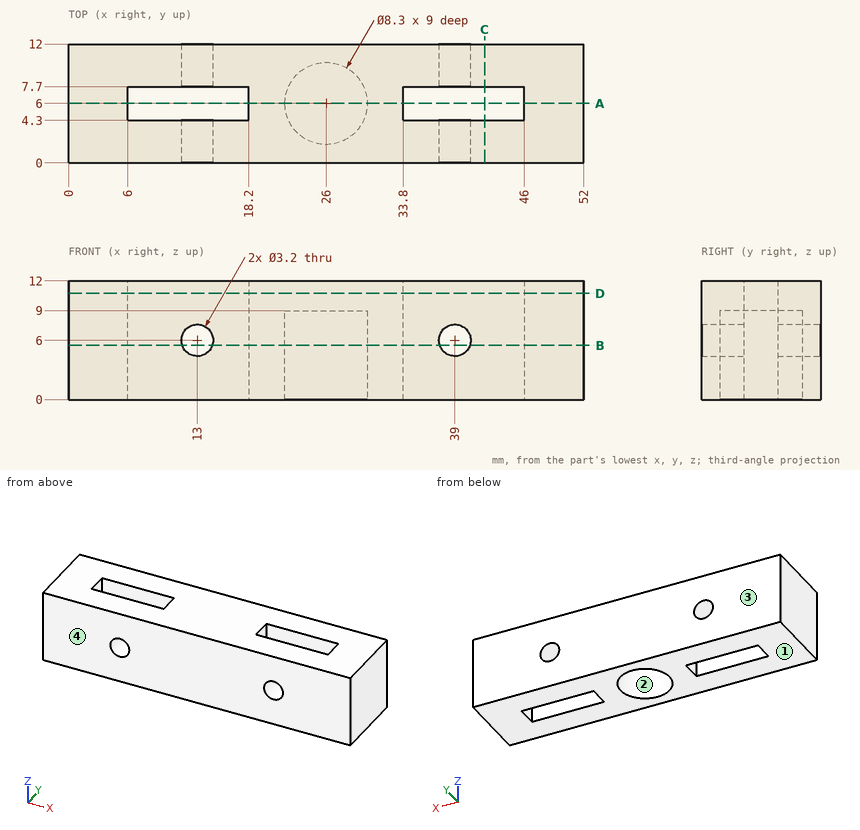
Input: dimensioned drawing with shaded views. Units: mm. Origin: part minimum x, y, z. Round coordinates to 2 decimals unless told otherwise and drop trailing zeros. Order: outer loops, then holes, each group sorted by start corner. A loop starts at its lowest first (then second) coordinate and runs counter-clockwise, first axis right, second up.
1. Cut plane C-C, the plane x = 42. Output: boundary loops of the cut face in (y, z).
The answers:
outline: (0, 0) - (4.3, 0) - (4.3, 12) - (0, 12) - close; (7.7, 0) - (12, 0) - (12, 12) - (7.7, 12) - close
2. Material intervals for line 1 (X direction, y = 4.5, z = 11); line 2 (X direction, y = 5.75, z = 1.75); line 3 (Z direction, x = 39, y = 3.45), sorted ascending.
The answers:
line 1: x = 0 to 6, 18.2 to 33.8, 46 to 52
line 2: x = 0 to 6, 18.2 to 21.86, 30.14 to 33.8, 46 to 52
line 3: z = 0 to 4.4, 7.6 to 12
3. Pin query (flat end, axial travel): P1, Ø4, axis at x = 25.5, y = 6, coming from the -Z side. Return the tip coordinate at first contact, or that it passes through.
The answers:
P1: stops at z = 9
4. Mould query, pull axis Y, two halves, no side actions, for the marked faces 1, 2, 3 and 4. Classes: released by +Y, released by -Y, zero draft, split by the parting line, or undercut.
The answers:
face 1: zero draft
face 2: undercut
face 3: released by +Y
face 4: released by -Y
5. Cut plane A-A, the plane y = 6. Output: boundary loops of the cut face in (x, z).
The answers:
outline: (0, 0) - (6, 0) - (6, 12) - (0, 12) - close; (18.2, 0) - (21.85, 0) - (21.85, 9) - (30.15, 9) - (30.15, 0) - (33.8, 0) - (33.8, 12) - (18.2, 12) - close; (46, 0) - (52, 0) - (52, 12) - (46, 12) - close
6. Cut plane D-D, the plane z = 10.75. Output: boundary loops of the cut face in (x, y).
The answers:
outline: (0, 0) - (52, 0) - (52, 12) - (0, 12) - close; hole (6, 4.3) - (18.2, 4.3) - (18.2, 7.7) - (6, 7.7) - close; hole (33.8, 4.3) - (46, 4.3) - (46, 7.7) - (33.8, 7.7) - close
7. Cut plane B-B, the plane z = 5.5. State how many separate pieces and enclosed holes the cut face has, then the cut area to 3 significant figures.
The answers:
separate pieces: 3
enclosed holes: 1
area: 435 mm2
